from build123d import *

# Parameters (mm, degrees)
F0_W      = 127
F0_H      = 25.4
F1_DEPTH  = 6.35
F2_W      = 19.304
F2_H      = 3.81
F3_DEPTH  = 38.1
F4_W      = 3.048
F4_H      = 5.588
F5_DEPTH  = 6.351
F6_W      = 3.048
F6_H      = 5.588
F7_DEPTH  = 6.351
F8_W      = 4.572
F8_H      = 6.858
F8_W_2    = 3.048
F8_H_2    = 5.588
F9_DEPTH  = 4.445
F10_W     = 5.08
F10_H     = 25.4
F11_DEPTH = 19.05
F12_W     = 5.08
F12_H     = 25.4
F13_DEPTH = 19.05
F14_R     = 2.54
F15_DEPTH = 5.081
F16_R     = 5.08
F17_W     = 154.94
F17_H     = 5.08
F18_DEPTH = 12.7
F19_R     = 12.69999
F20_W     = 25.4
F20_H     = 39.37
F21_DEPTH = 12.7
F22_W     = 25.4
F22_H     = 12.7
F23_DEPTH = 12.7
F25_DEPTH = 38.101
F26_R     = 7.62


# Not quite as in the source:
# - a fillet or chamfer is up to 0.001 mm smaller than in the source, because OpenCascade refuses the exact size


with BuildPart() as f1:
    # F0 (on Front) → F1 (new body)
    with BuildSketch(Plane.XZ):
        with Locations((-63.5, 12.7)):
            Rectangle(F0_W, F0_H)
    extrude(amount=F1_DEPTH)

    # F2 (on face) → F3 (join)
    with BuildSketch(Plane.XZ.offset(6.35)):
        Polygon((-121.92, 25.4), (-127, 25.4), (-127, 0), (-121.92, 0), (-121.92, 21.59), align=None)
        with Locations((-112.268, 23.495)):
            Rectangle(F2_W, F2_H)
        Polygon((-97.536, 25.4), (-102.616, 25.4), (-102.616, 21.59), (-102.616, 0), (-97.536, 0), (-97.536, 21.59), align=None)
        with Locations((-87.884, 23.495)):
            Rectangle(F2_W, F2_H)
        Polygon((-73.152, 25.4), (-78.232, 25.4), (-78.232, 21.59), (-78.232, 0), (-73.152, 0), (-73.152, 21.59), align=None)
        with Locations((-63.5, 23.495)):
            Rectangle(F2_W, F2_H)
        Polygon((-48.768, 25.4), (-53.848, 25.4), (-53.848, 21.59), (-53.848, 0), (-48.768, 0), (-48.768, 21.59), align=None)
        with Locations((-39.116, 23.495)):
            Rectangle(F2_W, F2_H)
        Polygon((-24.384, 25.4), (-29.464, 25.4), (-29.464, 21.59), (-29.464, 0), (-24.384, 0), (-24.384, 21.59), align=None)
        with Locations((-14.732, 23.495)):
            Rectangle(F2_W, F2_H)
        Polygon((0, 25.4), (-5.08, 25.4), (-5.08, 21.59), (-5.08, 0), (0, 0), align=None)
    extrude(amount=F3_DEPTH)

    # F4 (on face) → F5 (cut, through all)
    with BuildSketch(Plane.XZ.offset(6.35)):
        with Locations((-14.732, 8.636)):
            Rectangle(F4_W, F4_H)
    extrude(amount=-F5_DEPTH, mode=Mode.SUBTRACT)

    # F6 (on face) → F7 (cut, through all)
    with BuildSketch(Plane.XZ.offset(6.35)):
        with Locations((-39.116, 8.636)):
            Rectangle(F6_W, F6_H)
        with Locations((-63.5, 8.636)):
            Rectangle(F6_W, F6_H)
        with Locations((-87.884, 8.636)):
            Rectangle(F6_W, F6_H)
        with Locations((-112.268, 8.636)):
            Rectangle(F6_W, F6_H)
    extrude(amount=-F7_DEPTH, mode=Mode.SUBTRACT)

    # F8 (on face) → F9 (cut)
    with BuildSketch(Plane(origin=(0, 0, 0), x_dir=(-1, 0, 0), z_dir=(0, 1, 0))):
        with Locations((14.732, 8.636)):
            Rectangle(F8_W, F8_H)
        with Locations((14.732, 8.636)):
            Rectangle(F8_W_2, F8_H_2, mode=Mode.SUBTRACT)
        with Locations((112.268, 8.636)):
            Rectangle(F8_W, F8_H)
        with Locations((112.268, 8.636)):
            Rectangle(F8_W_2, F8_H_2, mode=Mode.SUBTRACT)
        with Locations((87.884, 8.636)):
            Rectangle(F8_W, F8_H)
        with Locations((87.884, 8.636)):
            Rectangle(F8_W_2, F8_H_2, mode=Mode.SUBTRACT)
        with Locations((63.5, 8.636)):
            Rectangle(F8_W, F8_H)
        with Locations((63.5, 8.636)):
            Rectangle(F8_W_2, F8_H_2, mode=Mode.SUBTRACT)
        with Locations((39.116, 8.636)):
            Rectangle(F8_W, F8_H)
        with Locations((39.116, 8.636)):
            Rectangle(F8_W_2, F8_H_2, mode=Mode.SUBTRACT)
    extrude(amount=-F9_DEPTH, mode=Mode.SUBTRACT)

    # F10 (on face) → F11 (join)
    with BuildSketch(Plane.YZ):
        with Locations((-41.91, 12.7)):
            Rectangle(F10_W, F10_H)
    extrude(amount=F11_DEPTH)

    # F12 (on face) → F13 (join)
    with BuildSketch(Plane(origin=(-127, 0, 0), x_dir=(0, -1, 0), z_dir=(-1, 0, 0))):
        with Locations((41.91, 12.7)):
            Rectangle(F12_W, F12_H)
    extrude(amount=F13_DEPTH)

    # F14 (on face) → F15 (cut, through all)
    with BuildSketch(Plane(origin=(0, -39.37, 0), x_dir=(-1, 0, 0), z_dir=(0, 1, 0))):
        with Locations((-12.7, 12.7)):
            Circle(F14_R)
        with Locations((139.7, 12.7)):
            Circle(F14_R)
    extrude(amount=-F15_DEPTH, mode=Mode.SUBTRACT)

    # F16
    f16_edges = [f1.edges().sort_by_distance(p)[0] for p in [
        (19.05, -41.91, 0),
        (19.05, -41.91, 25.4),
        (-146.05, -41.91, 0),
        (-146.05, -41.91, 25.4),
        (-127, 0, 12.7),
        (0, 0, 12.7),
    ]]
    fillet(f16_edges, radius=F16_R)

    # F17 (on face) → F18 (join)
    with BuildSketch(Plane.XY.offset(25.4)):
        with Locations((-63.5, -41.91)):
            Rectangle(F17_W, F17_H)
    extrude(amount=F18_DEPTH)

    # F19 (radius 12.7 in the source; OpenCascade refuses exactly that, so slightly less here)
    f19_edges = [f1.edges().sort_by_distance(p)[0] for p in [
        (13.97, -41.91, 38.1),
        (-140.97, -41.91, 38.1),
    ]]
    fillet(f19_edges, radius=F19_R)

    # F20 (on face) → F21 (join)
    with BuildSketch(Plane.XY.offset(25.4)):
        with Locations((-63.5, -19.685)):
            Rectangle(F20_W, F20_H)
    extrude(amount=F21_DEPTH)

    # F22 (on face) → F23 (join)
    with BuildSketch(Plane(origin=(0, 0, 0), x_dir=(-1, 0, 0), z_dir=(0, 1, 0))):
        with Locations((63.5, 31.75)):
            Rectangle(F22_W, F22_H)
    extrude(amount=F23_DEPTH)

    # F24 (on face) → F25 (cut, through all)
    with BuildSketch(Plane.XY.offset(38.1)):
        with BuildLine():
            ThreePointArc((-55.88, 0), (-63.5, 7.62), (-71.12, 0))
            Line((-71.12, 0), (-55.88, 0))
        make_face()
    extrude(amount=-F25_DEPTH, mode=Mode.SUBTRACT)

    # F26
    f26_edges = [f1.edges().sort_by_distance(p)[0] for p in [
        (-50.8, 12.7, 31.75),
        (-76.2, 12.7, 31.75),
    ]]
    fillet(f26_edges, radius=F26_R)


solid = f1.part
Work out the finished part from the listing and answer in its coordinate system (mm). A direction names the side the tool comes from. Coordinates: 2 decimals unless noted, no trailing zeros. Loops run counter-clockwise (first coordinate to the right, second up) from the corner with the lowest first, then second, coordinate; pieces in that order, holes last. Notation, with made-up numbers: M 10.25,84.5 L 65.25,84.5 A19 ccw 65.25,116.5 Z; hole C -25,44 d7. An arc over 180 degrees is marked long. Answer in a Markdown table with one row per item. Add a question column.
1. Find section B-B, the plane y = -21. Write down the section's boundary in (x, z), then the cut area to 3 significant figures.
2. A tool of negligible diameter and unlimited length cuts with its end or side. For faces 5 (the flat face through (-112, -2, 5.207)), 6 (the flat face through (-112, -25, 21.59)), 7 (the cylindrical face through (-137.83, -41.87, 14.42)), from which of +Z, -Z, +X, -X, +Y, -Y can it reach the whole face along a straight path? Write none if from no direction.
3. Consider L1, parallel to X at y = -13.5, z = 20; L2, parallel to Y at x = -119, z = 21; L3, parallel to Y at x = -57.5, z = 29. Determine where each line is inside the solid, lowest interval first.
4. Find section C-C, the plane x = -21. Write down the section's boundary in (y, z).
5. Find section A-A, the plane x = -63.5. Write down the section's boundary in (y, z) (3 decimals).
6. Flat-ended cylindrical pins translate along their axes: P1, Ø5, axis at y = -11, z = 5.5, coming from the +X side; P2, Ø1, axis at x = -15, y = -5, coming from the +Z side; P3, Ø1.3, axis at y = -2, z = 9.5, coming from the +X side. Find the tip coordinate at first contact, or state that the pin passes through.
7. The mould has two halves that part along X. Classify faces 1 (the cylindrical face through (-144.522, -41.946, 1.449)), 2 (the flat face through (-17.018, -2, 9)), 3 (the cylindrical face through (17.522, -41.874, 23.951)), 4 (the flat face through (-97.536, -25, 11)): pulls with the +X half, pulls with the -X half, needs draft (parallel to the pull), parting line crosses it, or undercut.
8. Find section D-D, the plane y = -2. Write down the section's boundary in (x, z) (3 decimals), then the cut area to 3 significant figures.
Reported:
| question | item | result |
|---|---|---|
| 1 | outline | M -127,0 L -121.92,0 L -121.92,21.59 L -102.62,21.59 L -102.62,0 L -97.54,0 L -97.54,21.59 L -78.23,21.59 L -78.23,0 L -73.15,0 L -73.15,21.59 L -53.85,21.59 L -53.85,0 L -48.77,0 L -48.77,21.59 L -29.46,21.59 L -29.46,0 L -24.38,0 L -24.38,21.59 L -5.08,21.59 L -5.08,0 L 0,0 L 0,25.4 L -50.8,25.4 L -50.8,38.1 L -76.2,38.1 L -76.2,25.4 L -127,25.4 Z |
| 1 | area | 1,460 mm^2 |
| 2 | face 5 | +Y |
| 2 | face 6 | -Z, -Y |
| 2 | face 7 | +Y, -Y |
| 3 | L1 | x = -127 to -121.92, -102.62 to -97.54, -78.23 to -73.15, -53.85 to -48.77, -29.46 to -24.38, -5.08 to 0 |
| 3 | L2 | y = -6.35 to 0 |
| 3 | L3 | y = -44.45 to 0, 4.7 to 12.64 |
| 4 | outline | M -44.45,21.59 L -6.35,21.59 L -6.35,0 L 0,0 L 0,25.4 L -39.37,25.4 L -39.37,38.1 L -44.45,38.1 Z |
| 5 | outline | M -44.45,21.59 L -6.35,21.59 L -6.35,11.43 L -4.445,11.43 L -4.445,12.065 L 0,12.065 L 0,38.1 L -44.45,38.1 Z; M -6.35,0 L 0,0 L 0,5.207 L -4.445,5.207 L -4.445,5.842 L -6.35,5.842 Z; M 7.62,25.4 L 12.7,25.4 L 12.7,38.1 L 7.62,38.1 Z |
| 6 | P1 | stops at x = 0 |
| 6 | P2 | stops at z = 25.4 |
| 6 | P3 | stops at x = -0.62 |
| 7 | face 1 | pulls with the -X half |
| 7 | face 2 | undercut |
| 7 | face 3 | pulls with the +X half |
| 7 | face 4 | undercut |
| 8 | outline | M -125.96,0 L -1.04,0 L -1.04,25.4 L -50.8,25.4 L -50.8,38.1 L -76.2,38.1 L -76.2,25.4 L -125.96,25.4 Z; hole M -114.554,5.207 L -109.982,5.207 L -109.982,12.065 L -114.554,12.065 Z; hole M -90.17,5.207 L -85.598,5.207 L -85.598,12.065 L -90.17,12.065 Z; hole M -65.786,5.207 L -61.214,5.207 L -61.214,12.065 L -65.786,12.065 Z; hole M -41.402,5.207 L -36.83,5.207 L -36.83,12.065 L -41.402,12.065 Z; hole M -17.018,5.207 L -12.446,5.207 L -12.446,12.065 L -17.018,12.065 Z |
| 8 | area | 3,340 mm^2 |
